Part model, mm, in its own coordinate system. A direction names the side the tool comes from. Coordinates: 2 decimals unless noted, no trailing zeros. Write each loop counter-clockwise with the first axis right and the second up, starting at its lowest first coordinate (ties: lowest second). Pieces come first, ordered by that corner, then holes. Notation, with made-up numbers: (28.5, 3) -> (69.5, 3) arc R34 ccw to (69.5, 42) -> close; hole circle Ø10 at (64, 9). An arc over 180 degrees is marked (long way). Write item = value, one per line. Start each with the question number.
Q1. Tool access for faces 4 (the cylindrical face through (-294.97, -51.33, 166.74)), 5 (the flat face through (282.5, -99, -158)): list every direction of +Z, -Z, +X, -X, +Y, -Y with a clear straight run to the whole face (end or side of a thin tool).
Q2. Band-saw the part on C-C, the plane x = 80. List the corners of the cut face in (y, z), plus the area to 4 significant figures.
Q3. Pin check, flat tip, straight feed: P1, Ø18, axis at y = -47.5, z = 157.5, coming from the +X side. Stop position of the tip, or through.
Q4. Probe line 1 (Z direction, x = -294, y = -77); line 2 (X direction, y = -127.5, z = -155.5); line 3 (Y direction, x = -193, z = -164.5). List the from-to ranges inside material, lowest first.
Q5. Band-saw the part on B-B, the plane z = 30. List the corners of the cut face in (x, y), plus the area to 4 significant figures.
Q6. Pull direction X, two halves, no side cores. Call faces 1 (the cylindrical face through (285.03, -51.33, 166.74)), 2 (the cylindrical face through (60.476, 0.035, 25.664)), 3 (the flat face through (287.5, -96, 134)): released by +X, released by -X, zero draft, split by the parting line, or undercut.
Q7. Band-saw the part on D-D, the plane y = -47.5. Give the number of separate pieces and of enclosed holes in the cut face, plus the area to 3 significant figures.
Q8. Band-saw the part on A-A, the plane y = -171.5. List the corners of the cut face in (x, z), plus the area to 3 significant figures.
from build123d import *

# Parameters (mm, degrees)
SKETCH1_W               = 585
SKETCH1_H               = 395
SKETCH1_W_2             = 425
SKETCH1_H_2             = 235
BOSS_EXTRUDE1_DEPTH     = 2.5
SKETCH2_W               = 79.998803747
SKETCH2_H               = 200
BOSS_EXTRUDE2_DEPTH     = 5
MIRROR5_COPY_1_SKETCH_W = 79.998803747
MIRROR5_COPY_1_SKETCH_H = 200
MIRROR5_COPY_1_DEPTH    = 5
CUT_EXTRUDE2_DEPTH      = 649.257279172
CUT_EXTRUDE2_DEPTH_BACK = 649.257279172
SKETCH5_R               = 10
SKETCH7_W               = 425
SKETCH7_H               = 235
BOSS_EXTRUDE4_DEPTH     = 5
SKETCH8_R               = 20
CUT_EXTRUDE3_DEPTH      = 10


with BuildPart() as part:
    # Sketch1 → Boss-Extrude1 (new, symmetric)
    with BuildSketch(Plane(origin=(0, 0, 0), x_dir=(1, 0, 0), z_dir=(0, 1, 0))):
        with Locations((-5, 0)):
            Rectangle(SKETCH1_W, SKETCH1_H)
        with Locations((-5, 0)):
            Rectangle(SKETCH1_W_2, SKETCH1_H_2, mode=Mode.SUBTRACT)
    extrude(amount=BOSS_EXTRUDE1_DEPTH, both=True)

    # Sketch2 → Boss-Extrude2 (add)
    with BuildSketch(Plane.ZY.offset(297.5)):
        with Locations((-157.500598126, -97.5)):
            Rectangle(SKETCH2_W, SKETCH2_H)
    boss_extrude2 = extrude(amount=-BOSS_EXTRUDE2_DEPTH)

    # Mirror1: Boss-Extrude2 across plane
    add(boss_extrude2.mirror(Plane.XY))

    # Mirror5: Boss-Extrude2 across plane
    add(boss_extrude2.mirror(Plane(origin=(-5, 0, 0), x_dir=(0, 0, 1), z_dir=(1, 0, 0))))

    # Mirror5 copy 1 sketch → Mirror5 copy 1 (add)
    with BuildSketch(Plane(origin=(287.5, 0, 0), x_dir=(0, 0, -1), z_dir=(1, 0, 0))):
        with Locations((-157.500598126, -97.5)):
            Rectangle(MIRROR5_COPY_1_SKETCH_W, MIRROR5_COPY_1_SKETCH_H)
    extrude(amount=-MIRROR5_COPY_1_DEPTH)

    # Sketch5 → Cut-Extrude2 (cut, two sides: drawn at the far end of the back side and taken through both)
    with BuildSketch(Plane.ZY.offset(297.5).offset(-CUT_EXTRUDE2_DEPTH_BACK)):
        with Locations((-157.500598127, -17.5)):
            Circle(SKETCH5_R)
        with Locations((-157.500598127, -47.5)):
            Circle(SKETCH5_R)
        with Locations((-157.500598127, -77.5)):
            Circle(SKETCH5_R)
        with Locations((157.500598127, -17.5)):
            Circle(SKETCH5_R)
        with Locations((157.500598127, -47.5)):
            Circle(SKETCH5_R)
        with Locations((157.500598127, -77.5)):
            Circle(SKETCH5_R)
    extrude(amount=CUT_EXTRUDE2_DEPTH + CUT_EXTRUDE2_DEPTH_BACK, mode=Mode.SUBTRACT)

    # Sketch7 → Boss-Extrude4 (add)
    with BuildSketch(Plane(origin=(0, 2.5, 0), x_dir=(1, 0, 0), z_dir=(0, 1, 0))):
        with Locations((-5, 0)):
            Rectangle(SKETCH7_W, SKETCH7_H)
    extrude(amount=-BOSS_EXTRUDE4_DEPTH)

    # Sketch8 → Cut-Extrude3 (cut)
    with BuildSketch(Plane(origin=(0, 2.5, 0), x_dir=(1, 0, 0), z_dir=(0, 1, 0))):
        with Locations(Location((-80, 30, 0), (0, 0, 270))):
            Circle(SKETCH8_R)
        with Locations(Location((80, 30, 0), (0, 0, 270))):
            Circle(SKETCH8_R)
        with Locations(Location((80, -30, 0), (0, 0, 270))):
            Circle(SKETCH8_R)
        with Locations(Location((-80, -30, 0), (0, 0, 270))):
            Circle(SKETCH8_R)
    extrude(amount=-CUT_EXTRUDE3_DEPTH, mode=Mode.SUBTRACT)


solid = part.part
Ans:
q1.face_4 = +X, -X
q1.face_5 = +Z, -Z, -Y
q2.outline = (-2.5, -197.5) -> (2.5, -197.5) -> (2.5, -50) -> (-2.5, -50) -> close; (-2.5, -10) -> (2.5, -10) -> (2.5, 10) -> (-2.5, 10) -> close; (-2.5, 50) -> (2.5, 50) -> (2.5, 197.5) -> (-2.5, 197.5) -> close
q2.area = 1,575 mm2
q3.P1 = through
q4.line_1 = -197.5 to -167.49, -147.51 to -117.5, 117.5 to 147.51, 167.49 to 197.5
q4.line_2 = -297.5 to -292.5, 282.5 to 287.5
q4.line_3 = -2.5 to 2.5
q5.outline = (-297.5, -2.5) -> (-100, -2.5) -> (-100, 2.5) -> (-297.5, 2.5) -> close; (-60, -2.5) -> (60, -2.5) -> (60, 2.5) -> (-60, 2.5) -> close; (100, -2.5) -> (287.5, -2.5) -> (287.5, 2.5) -> (100, 2.5) -> close
q5.area = 2,525 mm2
q6.face_1 = zero draft
q6.face_2 = undercut
q6.face_3 = released by +X
q7.separate_pieces = 8
q7.enclosed_holes = 0
q7.area = 1,200 mm2
q8.outline = (-297.5, -197.5) -> (-292.5, -197.5) -> (-292.5, -117.5) -> (-297.5, -117.5) -> close; (-297.5, 117.5) -> (-292.5, 117.5) -> (-292.5, 197.5) -> (-297.5, 197.5) -> close; (282.5, -197.5) -> (287.5, -197.5) -> (287.5, -117.5) -> (282.5, -117.5) -> close; (282.5, 117.5) -> (287.5, 117.5) -> (287.5, 197.5) -> (282.5, 197.5) -> close
q8.area = 1,600 mm2
